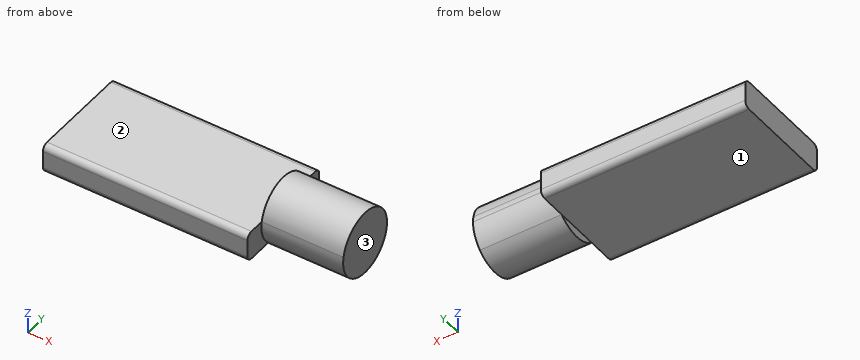
```python
from build123d import *

# Parameters (mm, degrees)
F0_W     = 35
F0_H     = 18
F1_DEPTH = 5
F3_DEPTH = 14
F4_R     = 1


with BuildPart() as f1:
    # F0 (on Top) → F1 (new body)
    with BuildSketch(Plane.XY):
        with Locations((17.5, 9)):
            Rectangle(F0_W, F0_H)
    extrude(amount=F1_DEPTH)

    # F2 (on face) → F3 (join)
    with BuildSketch(Plane.YZ.offset(35)):
        with BuildLine():
            Line((3.5916730868, 5), (14.4083269132, 5))
            ThreePointArc((14.4083269132, 5), (9, 9.5), (3.5916730868, 5))
        make_face()
        with BuildLine():
            ThreePointArc((12.7749172176, 0), (14.0503487353, 1.8219325879), (14.5, 4))
            ThreePointArc((14.5, 4), (14.4770337785, 4.502096593), (14.4083269132, 5))
            Line((14.4083269132, 5), (3.5916730868, 5))
            ThreePointArc((3.5916730868, 5), (3.7719034829, 2.2920752919), (5.2250827824, 0))
            Line((5.2250827824, 0), (12.7749172176, 0))
        make_face()
        with BuildLine():
            ThreePointArc((5.2250827824, 0), (9, -1.5), (12.7749172176, 0))
            Line((12.7749172176, 0), (5.2250827824, 0))
        make_face()
    extrude(amount=F3_DEPTH)

    # F4
    f4_edges = [f1.edges().sort_by_distance(p)[0] for p in [
        (17.5, 0, 5),
        (17.5, 18, 5),
        (17.5, 0, 0),
        (17.5, 18, 0),
    ]]
    fillet(f4_edges, radius=F4_R)


solid = f1.part
```
Model file for the job. Use its own axes, mm. Face numbers are marked on the shaded views. A direction names the side the tool comes from. Give positions to 0.01 mm unless a question says otherwise; leave off trailing zeros. Order: outer loops, then holes, each group sorted by start corner. A loop starts at its lowest first (then second) coordinate and runs counter-clockwise, first axis right, second up.
1) 3-axis set-ups, long thin cutter, end or side, ignore diameter. For the marked faces 1, 2 and 3: which of +Z, -Z, +X, -X, +Y, -Y reach the whole face in a straight line?
2) Saw through at A-A, the plane x = 30.5. Write the cut outline in (y, z).
3) Saw through at D-D, the plane x = 42. Write the cut outline in (y, z).
4) Pin check, flat tips, straight feed: pin 1 (1.5 mm diameter, centred on y = 2, z = 3.5, fed in from +X); pin 2 (3 mm diameter, centred on x = 9.5, y = 15.5, fed in from -Z); pin 3 (1.3 mm diameter, centred on y = 7, z = 7.5, fed in from -X). Stop position of each tip, or through.
5) Wall check: probe 1 along Z at (x, y) = (22, 10); probe 2 along X at (y, z) = (3, 1.25); probe 3 along X at (y, z) = (9.5, 7.5). Give the ranges that are in metal, low to high.
6) Saw through at B-B, the plane z = 2.75. Write the cut outline in (x, y).
7) Saw through at C-C, the plane y = 3. Write the cut outline in (x, z).
Computed:
1. face 1: -Z, -X, +Y, -Y
1. face 2: +Z, -X, +Y, -Y
1. face 3: +Z, -Z, +X, +Y, -Y
2. outline: (0, 1) arc R1 ccw to (1, 0) - (17, 0) arc R1 ccw to (18, 1) - (18, 4) arc R1 ccw to (17, 5) - (1, 5) arc R1 ccw to (0, 4) - close
3. outline: circle Ø11 at (9, 4)
4. pin 1: stops at x = 35
4. pin 2: stops at z = 0
4. pin 3: stops at x = 35
5. probe 1: z = 0 to 5
5. probe 2: x = 0 to 35
5. probe 3: x = 35 to 49
6. outline: (0, 0) - (35, 0) - (35, 3.64) - (49, 3.64) - (49, 14.36) - (35, 14.36) - (35, 18) - (0, 18) - close
7. outline: (0, 0) - (35, 0) - (35, 5) - (0, 5) - close
